Work out the finished part from the listing and answer in its coordinate system (mm). Face numbers are marked on the shaded views. A direction names the side the tool comes from. Round coordinates to 2 decimals unless told otherwise and drop trailing zeros. Write each loop counter-clockwise with the first axis right and the second up, starting at its lowest first coordinate (ties: lowest second). Pieces come first, ordered by that corner, then holes. Notation, with made-up numbers: (-34, -33) -> (0, -33) arc R25 cw to (0, -4) -> close; hole circle Ø7 at (1.5, 68.25). An arc over 180 degrees is marked (long way). One line per item, written item: value.
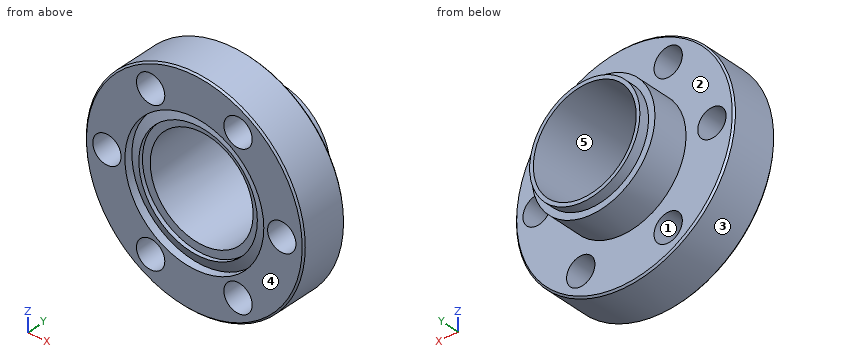
```python
from build123d import *

# Parameters (mm, degrees)
SKETCH2_R                 = 9.4996
BOSS_EXTRUDE1_DEPTH       = 5.461
SKETCH3_R                 = 8.509
BOSS_EXTRUDE2_DEPTH       = 1.524
M13_CLEARANCE_HOLE1_D     = 15.875
M13_CLEARANCE_HOLE1_DEPTH = 12.9286
M4_CLEARANCE_HOLE1_D      = 4.3688
M4_CLEARANCE_HOLE1_DEPTH  = 14.224
CHAMFER1_SIZE             = 0.254


with BuildPart() as part:
    # Sketch1 → Revolve1 (revolve)
    with BuildSketch(Plane(origin=(0, 0, 0), x_dir=(-1, 0, 0), z_dir=(0, 0, -1))):
        Polygon((-9.144, 1.2954), (0, 1.2954), (0, 7.239), (-16.637, 7.239), (-16.891, 6.985), (-16.891, 0), (-10.7188, 0), (-10.7188, 1.233580325), (-9.144, 0.6604), align=None)
    revolve(axis=Axis((0, 0, 0), (0, 1, 0)))

    # Sketch2 → Boss-Extrude1 (add)
    with BuildSketch(Plane(origin=(0, 7.239, 0), x_dir=(-1, 0, 0), z_dir=(0, 1, 0))):
        Circle(SKETCH2_R)
    extrude(amount=BOSS_EXTRUDE1_DEPTH)

    # Sketch3 → Boss-Extrude2 (add)
    with BuildSketch(Plane(origin=(0, 12.7, 0), x_dir=(-1, 0, 0), z_dir=(0, 1, 0))):
        Circle(SKETCH3_R)
    extrude(amount=BOSS_EXTRUDE2_DEPTH)

    # M13 Clearance Hole1
    with Locations(Plane(origin=(0, 14.224, 0), x_dir=(1, 0, 0), z_dir=(0, 1, 0))):
        with Locations((0, 0)):
            Hole(M13_CLEARANCE_HOLE1_D / 2, depth=M13_CLEARANCE_HOLE1_DEPTH)

    # M4 Clearance Hole1
    with Locations(Plane(origin=(0, 0, 0), x_dir=(-1, 0, 0), z_dir=(0, -1, 0))):
        with Locations((-13.4874, 0), (-6.7437, -11.680431031), (6.7437, -11.680431031), (13.4874, 0), (6.7437, 11.680431031), (-6.7437, 11.680431031)):
            Hole(M4_CLEARANCE_HOLE1_D / 2, depth=M4_CLEARANCE_HOLE1_DEPTH)

    # Chamfer1
    chamfer1_edges = [part.edges().sort_by_distance(p)[0] for p in [
        (-16.891, 0, 0),
    ]]
    chamfer(chamfer1_edges, length=CHAMFER1_SIZE)


solid = part.part
```
(1) Find section B-B on y = 2.5. Give the vertices of the cut face in (x, z) (1 decimal), plus the area to 3 significant figures.
Reported:
outline: circle Ø33.8 at (0, 0); hole circle Ø4.4 at (-13.5, 0); hole circle Ø4.4 at (-6.7, -11.7); hole circle Ø4.4 at (-6.7, 11.7); hole circle Ø15.9 at (0, 0); hole circle Ø4.4 at (6.7, -11.7); hole circle Ø4.4 at (6.7, 11.7); hole circle Ø4.4 at (13.5, 0)
area: 608 mm2
(2) A tool of negligible diameter and unlimited length cuts with its end or side. For the marked faces 1 and 2, from which of +Z, -Z, +X, -X, +Y, -Y can it reach the whole face along a straight path? Write none if from no direction.
Reported:
face 1: +Y, -Y
face 2: +Y
(3) Find section C-C on z = 0. Give the number of separate pieces and of enclosed holes in the cut face, plus the area to 3 significant figures.
Reported:
separate pieces: 4
enclosed holes: 0
area: 78.9 mm2
(4) For a pull along Z with two mould halves and no side action, classify the marked faces 3, 4 and 5 as pulls with the +Z half, pulls with the -Z half, needs draft (parallel to the pull), parting line crosses it, or undercut.
Reported:
face 3: parting line crosses it
face 4: needs draft
face 5: undercut
(5) Flat-ended cylindrical pins translate along their axes: pin 1 Ø6 at (x, y) = (5.5, 11) entering from +Z; pin 2 Ø12 at (x, z) = (12, 1.5) entering from -Y; pin 3 Ø5.5 at (x, z) = (6.74, 11.68) entering from +Y; pin 4 Ø2 at (x, y) = (-4, 6) entering from -Z. Find the tip coordinate at first contact, or state that the pin passes through.
Reported:
pin 1: stops at z = 9.16
pin 2: stops at y = 0
pin 3: stops at y = 7.24
pin 4: stops at z = -16.62
(6) Find section D-D on y = 10.5. Give the vertices of the cut face in (x, z) (1 decimal).
Reported:
outline: circle Ø19 at (0, 0); hole circle Ø15.9 at (0, 0)
(7) Consider probe 1 along X at (y, z) = (4, 1); probe 2 along X at (y, z) = (2, 2); probe 3 along X at (y, z) = (1, -12.5). Determine where each line is inside the solid, lowest interval first.
Reported:
probe 1: x = -16.86 to -15.43, -11.55 to -7.87, 7.87 to 11.55, 15.43 to 16.86
probe 2: x = -16.77 to -14.37, -12.61 to -7.68, 7.68 to 12.61, 14.37 to 16.77
probe 3: x = -11.36 to -8.77, -4.72 to 4.72, 8.77 to 11.36
